The listing builds one solid part. Answer for the finished solid, in the listing's coordinates (mm). Coordinates: 2 decimals unless noted, no trailing zeros.
Autodesk Inventor part; units mm, degrees
ref_plane "YZ Plane" through (0, 0, 0) normal (1, 0, 0) x (0, 1, 0)
ref_plane "XZ Plane" through (0, 0, 0) normal (0, 1, 0) x (-1, 0, 0)
ref_plane "XY Plane" through (0, 0, 0) normal (0, 0, 1) x (1, 0, 0)
sketch "Sketch1" plane through (0, 0, 0) normal (0, 1, 0) x (-1, 0, 0)
  line L0 (34.3448, 44.4205) -> (-185.3652, 44.4205)
  line L1 (-185.3652, 44.4205) -> (-185.3652, -16.5395)
  line L2 (-185.3652, -16.5395) -> (34.3448, -16.5395)
  line L3 (34.3448, -16.5395) -> (34.3448, 44.4205)
  point P0 (0, 0)
  dimension "d0" = 60.96
  dimension "d1" = 219.71
extrude "Extrusion1" add sketch "Sketch1" along normal blind 12.7
sketch "Sketch2" plane through (0, 12.7, 0) normal (0, 1, 0) x (1, 0, 0)
  line L0 (-34.3448, -44.4205) -> (185.3652, -44.4205)
  line L1 (185.3652, 16.5395) -> (-34.3448, 16.5395)
  line L2 (-34.3448, 16.5395) -> (-34.3448, -44.4205)
  line L3 (185.3652, -44.4205) -> (185.3652, 16.5395)
  point P0 (0, 0)
  point P1 (46.9352, -28.1137)
  point P2 (46.9352, 0.2327)
  point P3 (104.2884, 0.2327)
  point P4 (104.2884, -28.1137)
  dimension "d4" = 28.3464
  dimension "d5" = 0
  dimension "d6" = 0
  dimension "d7" = 16.3068
  dimension "d8" = 16.3068
  dimension "d9" = 57.3532
  dimension "d10" = 0
  dimension "d11" = 0
  dimension "d12" = 81.28
  dimension "d13" = 81.0768
hole "Hole1" at (46.9352, 12.7, 28.1137) at (46.9352, 12.7, -0.2327) at (104.2884, 12.7, -0.2327) at (104.2884, 12.7, 28.1137) direction (0, -1, 0) diameter 6.35 end through all countersink diameter 12.7 countersink angle 82
sketch "Sketch5" plane through (-34.3448, 0, -16.5395) normal (-1, 0, 0) x (0, 0, 1)
  line L0 (0, 0) -> (0, 12.7)
  line L1 (0, 12.7) -> (60.96, 12.7)
  point P0 (16.5395, 0)
  point P1 (54.605, 5.7736)
  point P2 (6.35, 5.08)
  dimension "d21" = 48.26
  dimension "d22" = 6.35
  dimension "d23" = 7.62
hole "Hole2" at (-34.3448, 5.7736, 38.0655) at (-34.3448, 5.08, -10.1895) direction (1, 0, 0) diameter 1.524 end through all
properties part number "TopPlate"
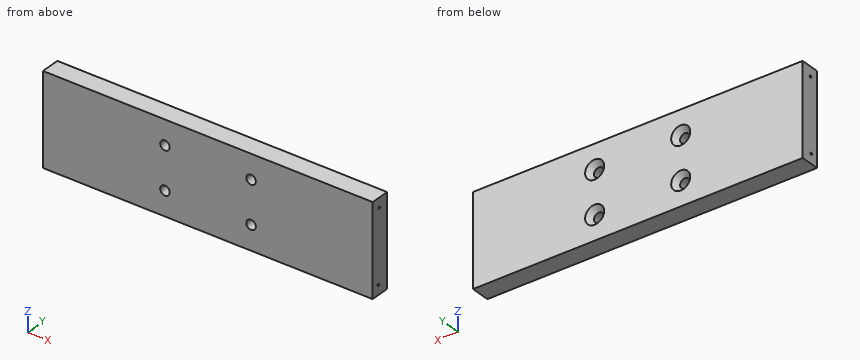
(1) Find the intervals of material crossed by probe 1 along X at (y, z) = (10.25, -3); probe 2 along Z at (x, y) = (92, 5.25); probe 3 along X at (y, z) = (5.75, -3), in increasing order.
(2) Section A-A, the plane z = 27.5 is taken. State how many separate pieces and enclosed holes the cut face has, plus the area to 3 significant figures.
(3) This flat-tipped pin is pushed along its axis until it touches: pin 1 (10 mm diameter, centred on x = 104.29, z = -0.23, fed in from -Y). Where does it stop, or does it pass through?
Solution:
1. probe 1: x = -34.34 to 43.75, 50.12 to 101.1, 107.47 to 185.37
1. probe 2: z = -16.54 to -10.93, -9.45 to 37.51, 38.62 to 44.42
1. probe 3: x = -34.34 to 45.38, 48.49 to 102.73, 105.84 to 185.37
2. separate pieces: 3
2. enclosed holes: 0
2. area: 2,610 mm2
3. pin 1: stops at y = 0
